Work out the finished part from the listing and answer in its coordinate system (mm). Face numbers are marked on the shaded views. A direction names the side the tool comes from. Round coordinates to 2 decimals unless told otherwise and drop trailing zeros. Loops run counter-clockwise (first coordinate to the right, second up) from the corner with the lowest first, then second, coordinate; pieces in that order, holes last.
from build123d import *

# Parameters (mm, degrees)
SKETCH011_W             = 19.95
SKETCH011_H             = 24.84
PAD002_DEPTH            = 3
POCKET008_DEPTH         = 12.421
POCKET008_DEPTH_BACK    = 12.421
SKETCH013_W             = 5
SKETCH013_H             = 0.56
POCKET009_DEPTH         = 12.421
POCKET009_DEPTH_BACK    = 12.421
BODY002_PLACEMENT_ANGLE = 270


with BuildPart() as part:
    # Sketch011 (on XY_Plane011 of Origin030) → Pad002 (new body)
    with BuildSketch(Plane.XY):
        with Locations((2.325, 0)):
            Rectangle(SKETCH011_W, SKETCH011_H)
    extrude(amount=PAD002_DEPTH)

    # Sketch012 (on XZ_Plane011 of Origin030) → Pocket008 (cut, two sides)
    with BuildSketch(Plane.XZ) as pocket008_sk:
        Polygon((-5.15, 0.866025), (-6.65, 0), (-3.65, 0), align=None)
    extrude(amount=-POCKET008_DEPTH, mode=Mode.SUBTRACT)
    extrude(pocket008_sk.sketch, amount=POCKET008_DEPTH_BACK, mode=Mode.SUBTRACT)

    # Sketch013 (on XZ_Plane011 of Origin030) → Pocket009 (cut, two sides)
    with BuildSketch(Plane.XZ) as pocket009_sk:
        with Locations((9.8, 0.28)):
            Rectangle(SKETCH013_W, SKETCH013_H)
    extrude(amount=-POCKET009_DEPTH, mode=Mode.SUBTRACT)
    extrude(pocket009_sk.sketch, amount=POCKET009_DEPTH_BACK, mode=Mode.SUBTRACT)


with BuildPart() as part_1:
    # Body002 placement: moved
    add(part.part.moved(Location((-1, 5.33, 42.62))).rotate(Axis((-1, 5.33, 42.62), (1, 0, 0)), BODY002_PLACEMENT_ANGLE))


solid = part_1.part
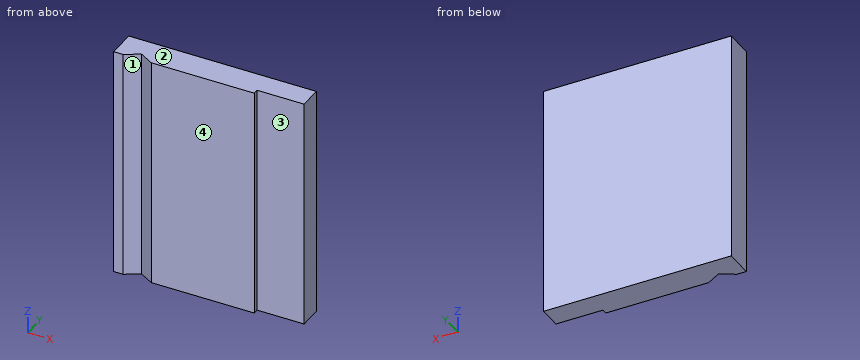
Item 1: Each of these flat-tipped pins is pushed along its axis until it touches: P1, Ø0.6, axis at y = 5.5, z = 44, coming from the +X side; P2, Ø5, axis at x = 9, z = 41.5, coming from the -Y side. Where does it stop, or does it pass through?
Item 2: For the marked faces 3 and 4, determine the directions among +Z, -Z, +X, -X, +Y, -Y from which every point of the face is accessible in a straight line to the end or side of a thin tool.
Item 3: Determine the mould class of the marked faces 1 and 2 for opening direction X: pulls with the +X half, pulls with the -X half, needs draft (parallel to the pull), parting line crosses it, or undercut.
Item 4: Straight lines are drawn through the part: line 1 (Y direction, x = 8.25, z = 31.5); line 2 (Y direction, x = -5.25, z = 33). For each, find the intervals that lie inside material, in ascending order.
Item 5: Section B-B, the plane x = -6.5 is taken. Give the vertices of the cut face in (y, z).
Item 6: Section A-A, the plane z = 34 is taken. Give the vertices of the cut face in (x, y), plus the area to 3 significant figures.
Answer below:
1. P1: stops at x = 6.3
1. P2: stops at y = 5.89
2. face 3: +Z, -Z, +X, -Y
2. face 4: +Z, -Z, +X, -X, -Y
3. face 1: undercut
3. face 2: needs draft
4. line 1: y = 5.89 to 8.33
4. line 2: y = 5.68 to 8.33
5. outline: (5.99, 30.2) - (8.33, 30.2) - (8.33, 55.04) - (5.99, 55.04) - close
6. outline: (-8.65, 5.33) - (-7.65, 5.33) - (-6.15, 6.2) - (-4.65, 5.33) - (6.3, 5.33) - (6.3, 5.89) - (11.3, 5.89) - (11.3, 8.33) - (-8.65, 8.33) - close
6. area: 55.8 mm2
